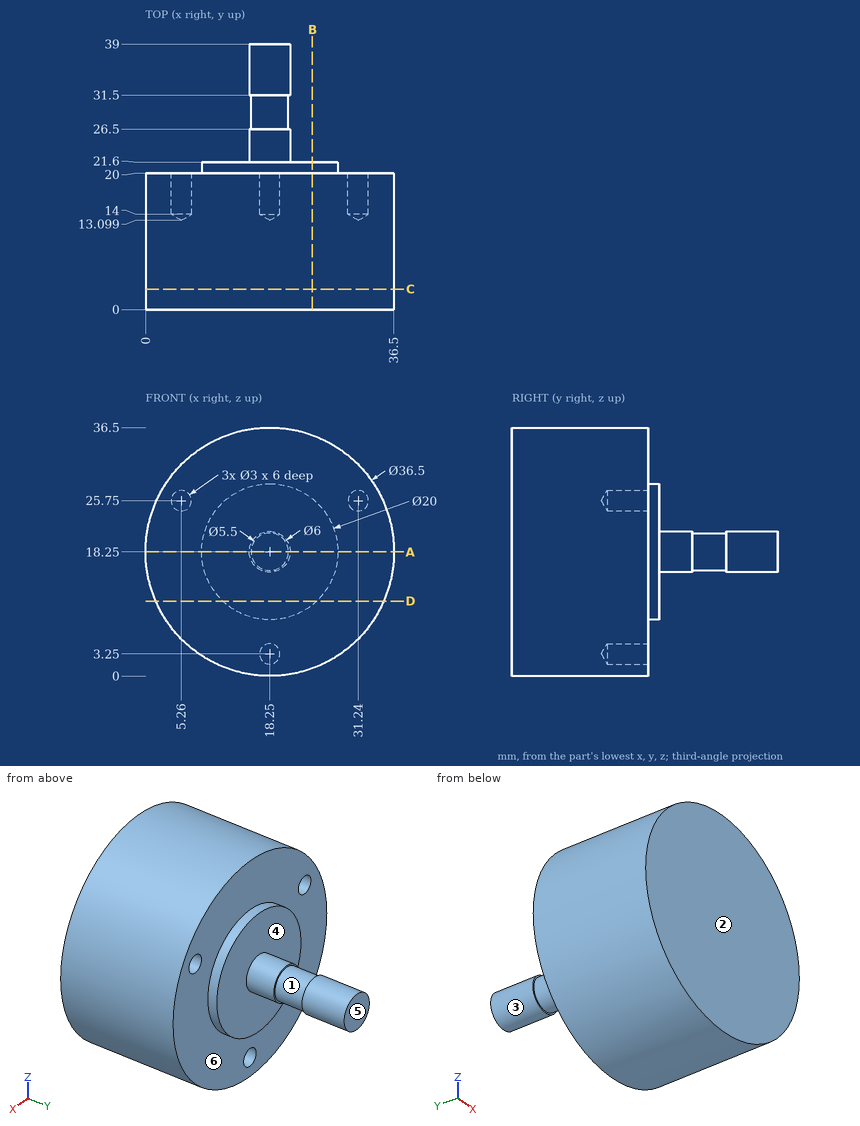
For this review, use the dimensioned drawing (mm, ordinates from the lowest corner) and the shaded views. A direction names the side the tool comes from. Round coordinates to 2 decimals unless told otherwise and drop trailing zeros. Write each loop counter-clockwise with the first axis right and the second up, starting at its lowest first coordinate (ties: lowest second). Pieces come first, ordered by that corner, then holes. Notation, with made-up numbers: (54, 37) - (88, 37) arc R32 ccw to (88, 67) - close; hole circle Ø5 at (0.25, 18.25). An arc over 180 degrees is marked (long way). Answer as a JSON object with one key per item and string values.
1. Tool access review of the marked faces 5 and 6: name each direction out of +Z, -Z, +X, -X, +Y, -Y from which nothing blocks a thin tool from reaching the whole face with its end or side.
Response values:
{"face 5": "+Z, -Z, +X, -X, +Y", "face 6": "+Y"}
2. To check wall thickness, follow line 1 along X through (y, z) = (15.3, 25.75); line 2 along Y through (x, z) = (13, 2.5); line 3 along Y through (x, z) = (27, 19). State the ranges of each line that lie inside material, in increasing order.
Response values:
{"line 1": "x = 1.61 to 3.76, 6.76 to 29.74, 32.74 to 34.89", "line 2": "y = 0 to 20", "line 3": "y = 0 to 21.6"}
3. We need section B-B on x = 24.5. Give the boundary of the cut face in (y, z).
Response values:
{"outline": "(0, 1.1) - (20, 1.1) - (20, 10.44) - (21.6, 10.44) - (21.6, 26.06) - (20, 26.06) - (20, 35.4) - (0, 35.4) - close"}
4. Draft analysis for pull direction Y (two halves, no side actions). For the marked faces 1, 2, 3 and 4, state which applies: +Y half, -Y half, draft (parallel to the pull), parting line (faces both ways), or undercut.
Response values:
{"face 1": "undercut", "face 2": "-Y half", "face 3": "draft", "face 4": "+Y half"}
5. We need section D-D on z = 11. Give the boundary of the cut face in (x, y).
Response values:
{"outline": "(1.5, 0) - (35, 0) - (35, 20) - (25.14, 20) - (25.14, 21.6) - (11.36, 21.6) - (11.36, 20) - (1.5, 20) - close"}
6. We need section A-A on z = 18.25. Give the boundary of the cut face in (x, y).
Response values:
{"outline": "(0, 0) - (36.5, 0) - (36.5, 20) - (28.25, 20) - (28.25, 21.6) - (21.25, 21.6) - (21.25, 26.5) - (21, 26.5) - (21, 31.5) - (21.25, 31.5) - (21.25, 39) - (15.25, 39) - (15.25, 31.5) - (15.5, 31.5) - (15.5, 26.5) - (15.25, 26.5) - (15.25, 21.6) - (8.25, 21.6) - (8.25, 20) - (0, 20) - close"}
7. We need section C-C on y = 3. Give the boundary of the cut face in (x, z).
Response values:
{"outline": "circle Ø36.5 at (18.25, 18.25)"}
8. For pin 1 Ø10 at (x, z) = (19.5, 28.5) entering from +Y; pin 2 Ø5 at (y, z) = (9.5, 24) entering from +X; pin 3 Ø2 at (y, z) = (10, 5) entering from -X, all flat-tipped, find the tip position at first contact; note any pin that passes through.
Response values:
{"pin 1": "stops at y = 21.6", "pin 2": "stops at x = 36.21", "pin 3": "stops at x = 4.72"}
